CAD build for the part. Positions are in the model's coordinates, mm. Coordinates: 2 decimals unless noted, no trailing zeros. Order: outer loops, then holes, each group sorted by start corner. A loop starts at its lowest first (then second) coordinate and runs counter-clockwise, first axis right, second up. Notation, with made-up numbers: M 33.5,75.5 L 47.5,75.5 A29 cw 47.5,106.5 Z; hole C 60.25,55.5 d10. An arc over 180 degrees is marked long. One line per item, written item: value.
from build123d import *

# Parameters (mm, degrees)
F0_R     = 130
F1_DEPTH = 5
F2_R     = 2.75
F2_R_2   = 4.25
F3_DEPTH = 5.001
F4_R     = 35
F5_DEPTH = 5.001


with BuildPart() as f1:
    # F0 (on Top) → F1 (new body)
    with BuildSketch(Plane.XY):
        Circle(F0_R)
    extrude(amount=F1_DEPTH)

    # F2 (on face) → F3 (cut, through all)
    with BuildSketch(Plane.XY.offset(5)):
        Circle(F2_R)
        with Locations((0, 115)):
            Circle(F2_R_2)
        with Locations((-99.592921, -57.5)):
            Circle(F2_R_2)
        with Locations((99.592921, -57.5)):
            Circle(F2_R_2)
    extrude(amount=-F3_DEPTH, mode=Mode.SUBTRACT)

    # F4 (on face) → F5 (cut, through all)
    with BuildSketch(Plane.XY.offset(5)):
        with Locations((-33.714593, 83.446547)):
            Circle(F4_R)
        with Locations((89.124126, -12.525579)):
            Circle(F4_R)
        with Locations((-55.409533, -70.920968)):
            Circle(F4_R)
    extrude(amount=-F5_DEPTH, mode=Mode.SUBTRACT)


solid = f1.part
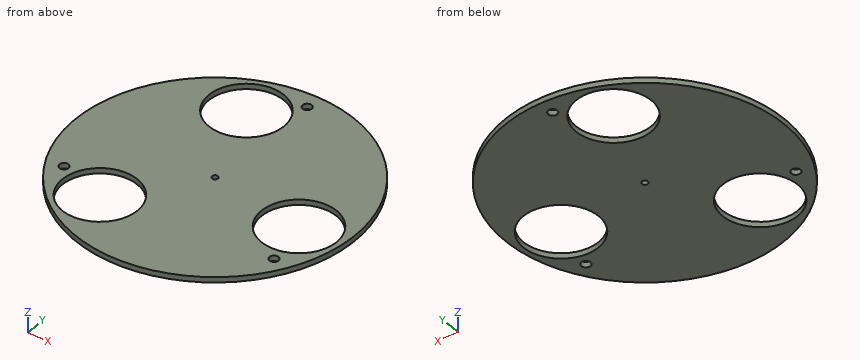
Q1. Slice it at D-D (z = 3.5). List the corners of the cut face in (x, y).
Recorded:
outline: C 0,0 d260; hole C -99.59,-57.5 d8.5; hole C -55.41,-70.92 d70; hole C -33.71,83.45 d70; hole C 0,115 d8.5; hole C 0,0 d5.5; hole C 89.12,-12.53 d70; hole C 99.59,-57.5 d8.5
Q2. Pin check, flat tips, straight feed: pin 1 Ø1.5 at (x, z) = (57, 2.5) entering from +Y; pin 2 Ø3 at (x, z) = (28, 1.5) entering from -Y; pin 3 Ø7.5 at (x, y) = (-99.59, -57.5) entering from -Z; pin 4 Ø2 at (x, z) = (31, 0.5) entering from -Y. Stop position of each tip, or through.
Recorded:
pin 1: stops at y = 117.2
pin 2: stops at y = -127.27
pin 3: passes through
pin 4: stops at y = -126.49
Q3. Slice it at B-B (x = -55). List the corners of the cut face in (y, z).
Recorded:
outline: M -117.79,0 L -105.92,0 L -105.92,5 L -117.79,5 Z; M -35.92,0 L 55.66,0 L 55.66,5 L -35.92,5 Z; M 111.23,0 L 117.79,0 L 117.79,5 L 111.23,5 Z
Q4. Slice it at A-A (y = 78.5). List the corners of the cut face in (x, z).
Recorded:
outline: M -103.62,0 L -68.36,0 L -68.36,5 L -103.62,5 Z; M 0.93,0 L 103.62,0 L 103.62,5 L 0.93,5 Z
Q5. Drill centre lines: line 1 along Y through (x, z) = (-58.5, 4.7); line 2 along X through (y, z) = (1, 0.95); line 3 along Y through (x, z) = (-64, 2.9). Where is each one in solid material? Low to high.
Recorded:
line 1: y = -116.09 to -105.78, -36.06 to 58.73, 108.16 to 116.09
line 2: x = -130 to -2.56, 2.56 to 56.84, 121.41 to 130
line 3: y = -113.15 to -104.85, -36.99 to 65.9, 100.99 to 113.15
Q6. Slice it at C-C (y = -57.5). List the corners of the cut face in (x, z), plus the area to 3 significant figures.
Recorded:
outline: M -116.59,0 L -103.84,0 L -103.84,5 L -116.59,5 Z; M -95.34,0 L -87.73,0 L -87.73,5 L -95.34,5 Z; M -23.08,0 L 95.34,0 L 95.34,5 L -23.08,5 Z; M 103.84,0 L 116.59,0 L 116.59,5 L 103.84,5 Z
area: 758 mm^2
